```python
from build123d import *


with BuildPart() as part:
    # Sketch 1 → Revolve 1 (revolve)
    with BuildSketch(Plane.XY, mode=Mode.PRIVATE) as revolve_1_sk:
        with BuildLine():
            Line((2.5, 2.5), (2.5, 3.5))
            Line((2.5, 3.5), (3, 4))
            Line((3, 4), (13.5, 4))
            Line((13.5, 4), (14, 3.5))
            Line((14, 3.5), (14, 1.5))
            Line((14, 1.5), (16, 1.5))
            Line((16, 1.5), (16, 1.2))
            Line((16, 1.2), (17, 1.2))
            Line((17, 1.2), (17, 2.5))
            Line((17, 2.5), (17.5, 3))
            Line((17.5, 3), (21.5, 3))
            Line((21.5, 3), (22, 2.5))
            Line((22, 2.5), (22, 0))
            Line((22, 0), (0, 0))
            ThreePointArc((0, 0), (0.732233047, 1.767766953), (2.5, 2.5))
        make_face()
    revolve(revolve_1_sk.sketch.rotate(Axis((22, 0, 0), (-1, 0, 0)), 270), axis=Axis((22, 0, 0), (-1, 0, 0)))


solid = part.part
```
CAD build for the part. Positions are in the model's coordinates, mm. A direction names the side the tool comes from. Coordinates: 2 decimals unless noted, no trailing zeros. Write each loop counter-clockwise with the first axis right and the second up, starting at its lowest first coordinate (ties: lowest second). Pieces come first, ordered by that corner, then holes.
(1) Drill centre lines: probe 1 along X at (y, z) = (-2.5, 2.25); probe 2 along X at (y, z) = (-0.5, 1.5); probe 3 along Y at (x, z) = (4, 1.75). Where is each one in solid material? Low to high.
(2) Cut at D-D, the plane x = 1.5. List the corners of the cut face in (y, z), and give its area (3 significant figures).
(3) Two-plate mould, pull along X, no slides. Class faces 1 (the face through (19.53, 0.9, 2.86)), 2 (the face through (17, 1, -1)), 3 (the face through (22, 0, 0)): +X half, -X half, draft (parallel to the pull), parting line (faces both ways), or undercut.
(4) 3-axis set-ups, long thin cutter, end or side, ignore diameter. For faces 4 (the face through (14, -2, 0)), 5 (the face through (8.324, -3.905, -0.867)), 6 (the face through (2.5, -2, -2)): which of +Z, -Z, +X, -X, +Y, -Y reach the whole face in a straight line?
(5) Flat gauge pins, fed straight in: pin 1 (1.5 mm diameter, centred on y = 0, z = -2, fed in from -X); pin 2 (4 mm diameter, centred on x = 19.5, z = 0, fed in from -Y); pin 3 (1 mm diameter, centred on x = 15.5, z = 1, fed in from -Y). Where does each tip first touch, or does it go through?
(6) Cut at A-A, the plane y = 0. List the corners of the cut face in (x, z), and give its area (3 significant figures).
(7) Cut at C-C, the plane x = 8. List the corners of the cut face in (y, z).
Geometry says:
1. probe 1: x = 2.5 to 14
1. probe 2: x = 0.56 to 14, 17 to 22
1. probe 3: y = -3.6 to 3.6
2. outline: circle Ø4.58 at (0, 0)
2. area: 16.5 mm2
3. face 1: draft
3. face 2: undercut
3. face 3: +X half
4. face 4: none
4. face 5: +X, -X
4. face 6: -X
5. pin 1: stops at x = 0.33
5. pin 2: stops at y = -3
5. pin 3: stops at y = -1.41
6. outline: (2.5, -3.5) - (3, -4) - (13.5, -4) - (14, -3.5) - (14, -1.5) - (16, -1.5) - (16, -1.2) - (17, -1.2) - (17, -2.5) - (17.5, -3) - (21.5, -3) - (22, -2.5) - (22, 2.5) - (21.5, 3) - (17.5, 3) - (17, 2.5) - (17, 1.2) - (16, 1.2) - (16, 1.5) - (14, 1.5) - (14, 3.5) - (13.5, 4) - (3, 4) - (2.5, 3.5) - (2.5, 2.5) arc R2.5 ccw to (2.5, -2.5) - close
6. area: 139 mm2
7. outline: circle Ø8 at (0, 0)
